For this review, use the dimensioned drawing (mm, ordinates from the lowest corner) and the shaded views. A direction names the side the tool comes from. Give positions to 0.01 mm unless a question says otherwise; leave off trailing zeros. Order: outer loops, then holes, each group sorted by start corner. A loop starts at its lowest first (then second) coordinate and runs counter-clockwise, first axis right, second up. Notation, with made-up numbers: M 71.25,-36 L 103.25,-36 A21 ccw 103.25,3 Z; hole C 47,40 d2. An arc over 180 degrees is marked long. One line per question, with ' | ' between items. Start each with the question number.
1. We need section B-B on x = 20.5. Write out the cut boundary in (y, z).
2. We need section A-A on z = 3.75. Write out the cut boundary in (x, y), then the cut area to 3 significant figures.
3. Insertion check: P1, Ø10, axis at x = 17.5, y = 7.5, coming from the -Z side; P2, Ø2, axis at y = 49.5, z = 5.5, coming from the +X side (1 decimal); P3, Ø8, axis at y = 21.5, z = 13.5, coming from the +X side; P4, Ø12, axis at y = 25.5, z = 4.5, coming from the -X side (1 decimal). Each pin has a flat end and moves straight along its axis. Give the tip position at first contact, or say it passes through.
4. The part is to be moulded in two halves that separate along Y. For the marked faces 1, 2 and 3, say which applies: +Y half, -Y half, draft (parallel to the pull), parting line (faces both ways), or undercut.
5. For the marked faces 4 and 5, list the 3-axis set-ups (+Z, -Z, +X, -X, +Y, -Y) from which the entire face can be reached by the end or side of a thin tool; tool diameter is ignored.
6. We need section C-C on y = 19. Write out the cut boundary in (x, z).
7. Wall thickness on L1, parallel to Y at x = 10.25, z = 5.5; L2, parallel to Z at x = 12.25, y = 47.5 (1 decimal); L3, parallel to Z at x = 14.5, y = 14 (1 decimal): over which ranges is each line inside the solid? List them lowest first.
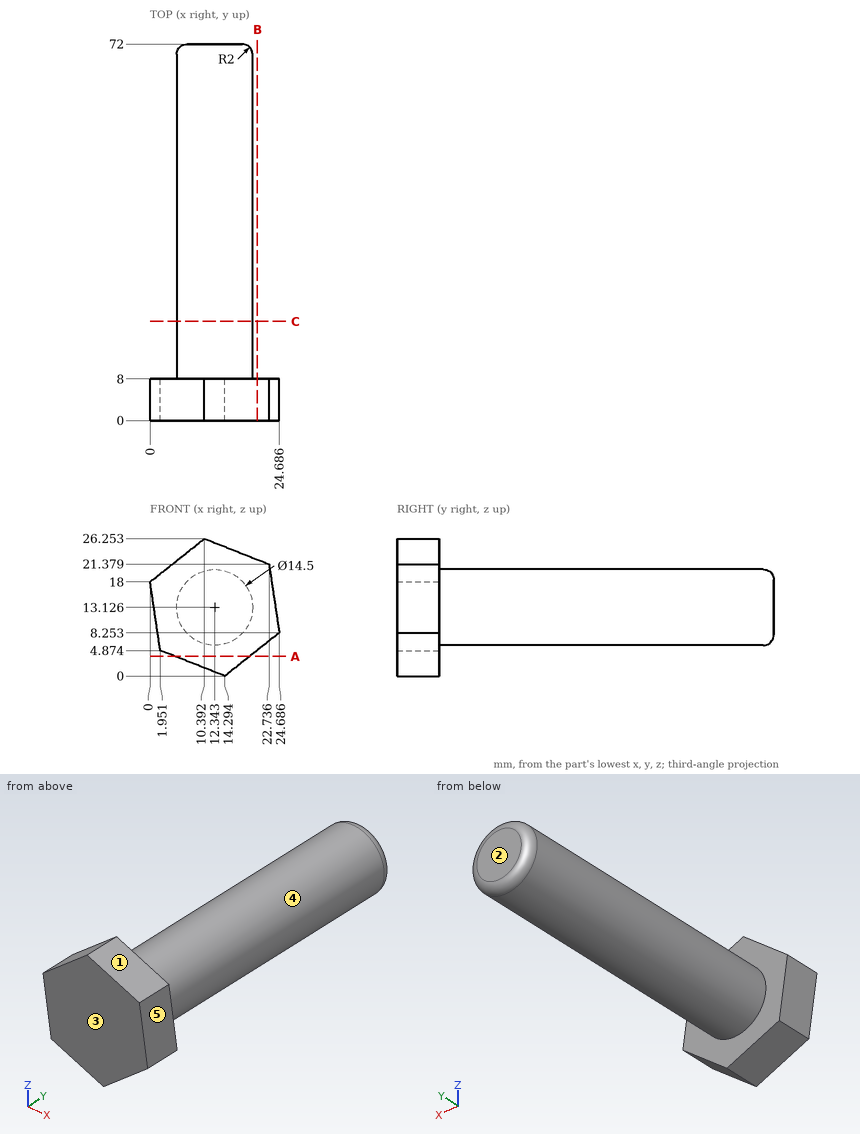
Entries:
1) outline: M 0,4.93 L 8,4.93 L 8,22.26 L 0,22.26 Z
2) outline: M 4.8,0 L 19.02,0 L 19.02,8 L 4.8,8 Z | area: 114 mm^2
3) P1: stops at z = 0 | P2: stops at x = 15.3 | P3: stops at x = 19.59 | P4: stops at x = 5.6
4) face 1: draft | face 2: +Y half | face 3: -Y half
5) face 4: +Y | face 5: +Z, +X, +Y, -Y
6) outline: C 12.34,13.13 d14.5
7) L1: y = 0 to 8 | L2: z = 5.9 to 20.4 | L3: z = 6.2 to 20
